Could you check a few things on this model? Use its own coordinates, in mm. Face numbers are marked on the shaded views. Round coordinates to 2 decimals unless told otherwise and drop trailing zeros. Write each loop counter-clockwise with the first axis right and the second up, starting at its lowest first coordinate (ties: lowest second). Pieces come first, ordered by that corner, then holes. Notation, with made-up numbers: (44.25, 33.5) -> (50.25, 33.5) arc R23 cw to (50.25, 47.5) -> close; hole circle Ø11 at (40.25, 9). An arc over 180 degrees is marked (long way). Answer as CSV lines item,"result". Start each with the question number.
Q1. Imagine slicing it at B-B on z = 12.5. Please give me the cut outline in (x, y), and give its area (3 significant figures).
Q2. Imagine slicing it at D-D on z = 23. Please give me the cut outline in (x, y).
Q3. If I drill on line 1 (Y direction, x = -0.5, z = 12.5); line 2 (Y direction, x = -26.5, z = 12.5); line 3 (Y direction, x = 0, z = 9), over which ranges is the centre line in solid material (lowest first)? Write a range as [from, to].
Q4. Will these pins go through, and if not, where does the flat tip stop? pin 1 Ø2.5 at (y, z) = (0, 12.5) entering from -X; pin 2 Ø5.5 at (y, z) = (0, 12.5) entering from +X.
Q5. Imagine slicing it at A-A on x = 0. Please give me the cut outline in (y, z), and give its area (3 significant figures).
Q6. Imagine slicing it at C-C on y = -25. Please give me the cut outline in (x, z).
Q7. If we mould it in two halves opening along X, with no side actions, what happens to the marked faces 1, 2 and 3? For each: pulls with the +X half, pulls with the -X half, needs draft (parallel to the pull), parting line crosses it, or undercut.
from build123d import *

# Parameters (mm, degrees)
BOSS_EXTRUDE1_DEPTH = 25
SKETCH2_R           = 2.1
CUT_EXTRUDE1_DEPTH  = 72.589105316


with BuildPart() as part:
    # Sketch1 → Boss-Extrude1 (new body)
    with BuildSketch(Plane.XY):
        with BuildLine():
            Line((-30, 0), (-20, 0))
            ThreePointArc((-20, 0), (0, 20), (20, 0))
            Line((20, 0), (30, 0))
            Line((30, 0), (30, 30))
            Line((30, 30), (-30, 30))
            Line((-30, 30), (-30, 0))
        make_face()
        with BuildLine():
            ThreePointArc((20, 0), (0, -20), (-20, 0))
            Line((-20, 0), (-30, 0))
            Line((-30, 0), (-30, -30))
            Line((-30, -30), (30, -30))
            Line((30, -30), (30, 0))
            Line((30, 0), (20, 0))
        make_face()
    extrude(amount=BOSS_EXTRUDE1_DEPTH)

    # Sketch2 → Cut-Extrude1 (cut, through all)
    with BuildSketch(Plane(origin=(30, 0, 0), x_dir=(0, 0, -1), z_dir=(1, 0, 0))):
        with Locations((-12.5, 25)):
            Circle(SKETCH2_R)
        with Locations((-12.5, -25)):
            Circle(SKETCH2_R)
        with Locations((-12.5, 0)):
            Circle(SKETCH2_R)
    extrude(amount=-CUT_EXTRUDE1_DEPTH, mode=Mode.SUBTRACT)


solid = part.part
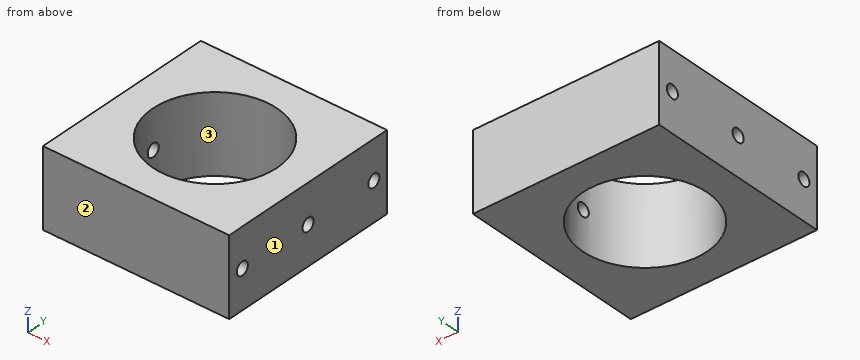
Checks:
1,outline,"(-30, -30) -> (30, -30) -> (30, -27.1) -> (-30, -27.1) -> close; (-30, -22.9) -> (30, -22.9) -> (30, -2.1) -> (19.89, -2.1) arc R20 cw to (-19.89, -2.1) -> (-30, -2.1) -> close; (-30, 2.1) -> (-19.89, 2.1) arc R20 cw to (19.89, 2.1) -> (30, 2.1) -> (30, 22.9) -> (-30, 22.9) -> close; (-30, 27.1) -> (30, 27.1) -> (30, 30) -> (-30, 30) -> close"
1,area,"1,760 mm^2"
2,outline,"(-30, -30) -> (30, -30) -> (30, 30) -> (-30, 30) -> close; hole circle Ø40 at (0, 0)"
3,line 1,"[-30, -27.1], [-22.9, -19.99], [19.99, 22.9], [27.1, 30]"
3,line 2,"[-30, -27.1], [-22.9, -2.1], [2.1, 22.9], [27.1, 30]"
3,line 3,"[-30, -20], [20, 30]"
4,pin 1,"through"
4,pin 2,"x = 30"
5,outline,"(-30, 0) -> (-20, 0) -> (-20, 25) -> (-30, 25) -> close; (20, 0) -> (30, 0) -> (30, 25) -> (20, 25) -> close; hole circle Ø4.2 at (-25, 12.5); hole circle Ø4.2 at (25, 12.5)"
5,area,"472 mm^2"
6,outline,"(-30, 0) -> (30, 0) -> (30, 10.4) -> (-30, 10.4) -> close; (-30, 14.6) -> (30, 14.6) -> (30, 25) -> (-30, 25) -> close"
7,face 1,"pulls with the +X half"
7,face 2,"needs draft"
7,face 3,"undercut"
